Drawing for the job (mm, zero at the part's lowest x, y, z). Round coordinates to 2 decimals unless told otherwise and drop trailing zeros. Write each loop counter-clockwise with the first axis right and the second up, starting at its lowest first coordinate (ties: lowest second). Pieces come first, ordered by that corner, then holes. Notation, with made-up numbers: (77, 22.5) -> (105, 22.5) arc R21 ccw to (105, 28.5) -> close; hole circle Ø8 at (79.25, 89). An arc over 180 degrees is marked (long way). Answer in a Markdown table with one row per item. Add a question column.
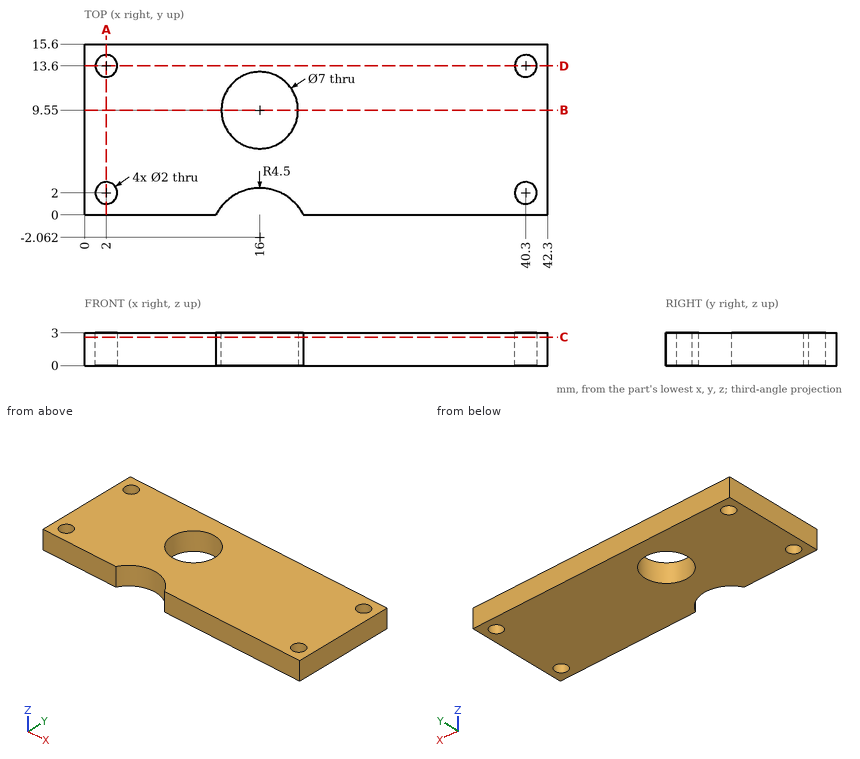
(1) Saw through at D-D (y = 13.6). List the corners of the cut face in (x, z), plus the area to 3 significant figures.
(2) Saw through at B-B (y = 9.55). List the corners of the cut face in (x, z).
(3) Saw through at A-A (x = 2). List the corners of the cut face in (y, z).
(4) Probe line 1 along Y through (x, z) = (2, 2.35); line 2 along Y through (x, z) = (16, 1.5); line 3 along X through (y, z) = (2.75, 1.9). List the from-to ranges inside material, lowest first.
(5) Saw through at C-C (z = 2.6). List the corners of the cut face in (x, y), plus the area to 3 significant figures.
Answer sheet:
| question | item | result |
|---|---|---|
| 1 | outline | (0, 0) -> (1, 0) -> (1, 3) -> (0, 3) -> close; (3, 0) -> (39.3, 0) -> (39.3, 3) -> (3, 3) -> close; (41.3, 0) -> (42.3, 0) -> (42.3, 3) -> (41.3, 3) -> close |
| 1 | area | 115 mm² |
| 2 | outline | (0, 0) -> (12.5, 0) -> (12.5, 3) -> (0, 3) -> close; (19.5, 0) -> (42.3, 0) -> (42.3, 3) -> (19.5, 3) -> close |
| 3 | outline | (0, 0) -> (1, 0) -> (1, 3) -> (0, 3) -> close; (3, 0) -> (12.6, 0) -> (12.6, 3) -> (3, 3) -> close; (14.6, 0) -> (15.6, 0) -> (15.6, 3) -> (14.6, 3) -> close |
| 4 | line 1 | y = 0 to 1, 3 to 12.6, 14.6 to 15.6 |
| 4 | line 2 | y = 2.44 to 6.05, 13.05 to 15.6 |
| 4 | line 3 | x = 0 to 1.34, 2.66 to 39.64, 40.96 to 42.3 |
| 5 | outline | (0, 0) -> (12, 0) arc R4.5 cw to (20, 0) -> (42.3, 0) -> (42.3, 15.6) -> (0, 15.6) -> close; hole circle Ø2 at (2, 2); hole circle Ø2 at (2, 13.6); hole circle Ø7 at (16, 9.55); hole circle Ø2 at (40.3, 2); hole circle Ø2 at (40.3, 13.6) |
| 5 | area | 595 mm² |
